Can you work these out from the model? Positions are in its coordinate system, mm. Coordinates: 2 decimals unless noted, no trailing zeros. Loops run counter-clockwise (first coordinate to the right, second up) from the corner with the lowest first, then second, coordinate; pieces in that order, holes last. Notation, with made-up numbers: (75.25, 73) -> (108.25, 73) arc R17 cw to (108.25, 86) -> close; hole circle Ø1 at (5.25, 7). An arc over 180 degrees is marked (long way). Use one line per item in the form item = value. Start each with the question number.
(1) Thinking about a two-plate mould opening in Z: for faces 1 (the flat face through (89.416, 2.465, -20.346)), 2 (the cylindrical face through (72.85, 2.46, -43.76)), 3 (the flat face through (36.98, 2.46, 46.02)), 4 (the cylindrical face through (100.1, 2.5, 30.5)), which applies, released by +Z, released by -Z, zero draft, split by the parting line, or undercut?
(2) Imagine slicing it at C-C (y = 1.5). State how many separate pieces and enclosed holes the cut face has, plus the area to 3 significant figures.
(3) Imagine slicing it at B-B (z = 20). List the corners of the cut face in (x, y) for me.
(4) Imagine slicing it at A-A (x = 18.25). List the corners of the cut face in (y, z) for me, plus the area to 3 significant figures.
(5) Imagine slicing it at D-D (z = -37.5). List the corners of the cut face in (x, y) for me, plus the area to 3 significant figures.
(6) I need wall thicknesses on line 1 (X direction, y = 2.5, z = 0); line 2 (X direction, y = 2.8, z = -3.5); line 3 (Z direction, x = 84, y = 0.3). Which ranges of each line are inside material? Lowest first, please. Write a range as [from, to].
(7) I'm going to push flat-ended pins straight in: pin 1 (2 mm diameter, centred on y = 2.5, z = -29.5, fed in from -X); pin 2 (1.5 mm diameter, centred on x = 30, y = 1.5, fed in from +Z). Where does each tip first touch, or does it pass through?
```python
from build123d import *

# Parameters (mm, degrees)
SKETCH1_R           = 25.1
SKETCH1_R_2         = 4
SKETCH1_R_3         = 1.5
SKETCH1_R_4         = 2.5
BOSS_EXTRUDE1_DEPTH = 5


with BuildPart() as part:
    # Sketch1 → Boss-Extrude1 (new body)
    with BuildSketch(Plane(origin=(0, 0, 0), x_dir=(1, 0, 0), z_dir=(0, 1, 0))):
        with BuildLine():
            Line((0, -47.5), (75, -44.5))
            ThreePointArc((75, -44.5), (100.341650726, -30.101348895), (100.945295539, -0.961067014))
            Line((100.945295539, -0.961067014), (77.559049402, 42.258960334))
            ThreePointArc((77.559049402, 42.258960334), (73.883135286, 46.090390077), (68.764033965, 47.5))
            Line((68.764033965, 47.5), (0, 47.5))
            ThreePointArc((0, 47.5), (-47.5, 0), (0, -47.5))
        make_face()
        with Locations(Location((75, -15, 0), (0, 0, 270))):
            Circle(SKETCH1_R, mode=Mode.SUBTRACT)
        with Locations(Location((0, 0, 0), (0, 0, 270))):
            Circle(SKETCH1_R_2, mode=Mode.SUBTRACT)
        with Locations(Location((88.688017257, 11.71100727, 0), (0, 0, 270))):
            Circle(SKETCH1_R_3, mode=Mode.SUBTRACT)
        with Locations(Location((56.591696316, 11.71100727, 0), (0, 0, 270))):
            Circle(SKETCH1_R_3, mode=Mode.SUBTRACT)
        with Locations(Location((56.591696316, -39.768646015, 0), (0, 0, 270))):
            Circle(SKETCH1_R_3, mode=Mode.SUBTRACT)
        with Locations(Location((18.25, 0, 0), (0, 0, 270))):
            Circle(SKETCH1_R_4, mode=Mode.SUBTRACT)
        with Locations(Location((-18.25, 0, 0), (0, 0, 270))):
            Circle(SKETCH1_R_4, mode=Mode.SUBTRACT)
        with Locations(Location((71.835494757, 42.654234046, 0), (0, 0, 270))):
            Circle(SKETCH1_R_3, mode=Mode.SUBTRACT)
        with Locations(Location((42.137334928, 43.5, 0), (0, 0, 270))):
            Circle(SKETCH1_R_3, mode=Mode.SUBTRACT)
        with Locations(Location((83.354686129, 23.142870245, 0), (0, 0, 270))):
            Circle(SKETCH1_R_3, mode=Mode.SUBTRACT)
        with Locations(Location((40.293422434, -41.885064382, 0), (0, 0, 270))):
            Circle(SKETCH1_R_3, mode=Mode.SUBTRACT)
    extrude(amount=BOSS_EXTRUDE1_DEPTH)


solid = part.part
```
Worked out:
q1.face_1 = released by -Z
q1.face_2 = undercut
q1.face_3 = released by +Z
q1.face_4 = split by the parting line
q2.separate_pieces = 1
q2.enclosed_holes = 11
q2.area = 10,100 mm2
q3.outline = (-43.08, 0) -> (50.4, 0) -> (50.4, 5) -> (-43.08, 5) -> close; (99.6, 0) -> (104.07, 0) -> (104.07, 5) -> (99.6, 5) -> close
q4.outline = (0, -47.5) -> (5, -47.5) -> (5, -2.5) -> (0, -2.5) -> close; (0, 2.5) -> (5, 2.5) -> (5, 46.77) -> (0, 46.77) -> close
q4.area = 446 mm2
q5.outline = (-29.15, 0) -> (80.13, 0) -> (80.13, 5) -> (-29.15, 5) -> close
q5.area = 546 mm2
q6.line_1 = [-47.5, -20.75], [-15.75, -4], [4, 15.75], [20.75, 54.88], [95.12, 100.43]
q6.line_2 = [-47.37, -1.94], [1.94, 58.04], [91.96, 98.53]
q6.line_3 = [-30.36, -24.5], [-21.79, -8.43], [38.43, 43.09]
q7.pin_1 = -38
q7.pin_2 = 46.33
